```python
from build123d import *

# Parameters (mm, degrees)
F0_R     = 381
F1_DEPTH = 762
F3_W     = 50
F3_H     = 50
F3_W_2   = 40
F3_H_2   = 40
F4_DEPTH = 30
F5_W     = 50
F5_H     = 50
F5_W_2   = 40
F5_H_2   = 40
F6_DEPTH = 30
F7_SIZE  = 24.99999


# Not quite as in the source:
# - a fillet or chamfer is up to 0.001 mm smaller than in the source, because OpenCascade refuses the exact size


with BuildPart() as f1:
    # F0 (on Top) → F1 (new body)
    with BuildSketch(Plane.XY):
        Circle(F0_R)
    extrude(amount=F1_DEPTH)


with BuildPart() as f4:
    # F3 (on Top) → F4 (new body)
    with BuildSketch(Plane.XY):
        Rectangle(F3_W, F3_H)
        Rectangle(F3_W_2, F3_H_2, mode=Mode.SUBTRACT)
    extrude(amount=F4_DEPTH)

    # F5 (on face) → F6 (join)
    with BuildSketch(Plane.XY.offset(30)):
        Rectangle(F5_W, F5_H)
        Rectangle(F5_W_2, F5_H_2, mode=Mode.SUBTRACT)
        Rectangle(F5_W_2, F5_H_2)
    extrude(amount=F6_DEPTH)

    # F7 (size 25 in the source; OpenCascade refuses exactly that, so slightly less here)
    f7_edges = [f4.edges().sort_by_distance(p)[0] for p in [
        (25, 0, 60),
        (0, 25, 60),
        (-25, 0, 60),
        (0, -25, 60),
    ]]
    chamfer(f7_edges, length=F7_SIZE)


solid = f4.part
```
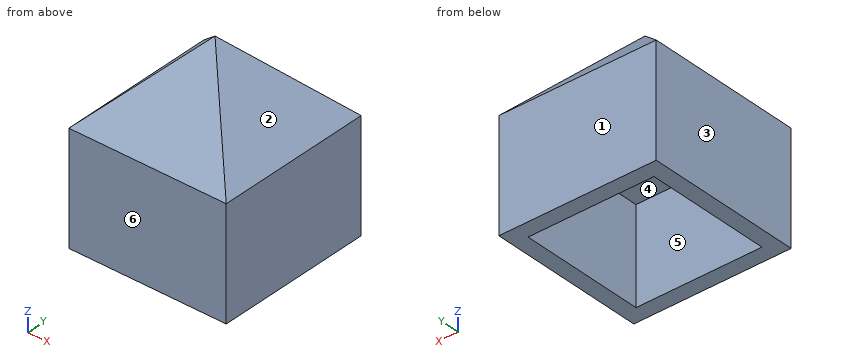
Source: CAD feature listing. Evaluate the final solid. Frame: model axes, mm. Face numbers are marked on the shaded views. A direction names the side the tool comes from. Give positions to 0.01 mm unless a question says otherwise; leave off trailing zeros. Write each loop counter-clockwise with the first axis right and the second up, starting at its lowest first coordinate (ties: lowest second). Pieces come first, ordered by that corner, then holes. Notation, with made-up numbers: (40, 47) - (79, 47) arc R14 cw to (79, 64) - close; hole circle Ø10 at (49.5, 71.25). An arc over 180 degrees is marked (long way). One line per item, written item: value. Start each with the question number.
Q1. Set-up query: the marked faces 5 and 6. Return all of +Z, -Z, +X, -X, +Y, -Y with unobstructed straight access to the full face (end or side cutting, diameter ignored); none if empty.
Q2. Material intervals for probe 1 along Y at (x, z) = (-16, 26.5); probe 2 along Z at (x, y) = (-16, 6.5), sorted ascending. Write a range as from..to.
Q3. Section query D-D, the plane z = 39. Return the cut outline in (x, y), then the cut area to 3 significant figures.
Q4. Section query A-A, the plane z = 12.5. Return the cut outline in (x, y), then the cut area to 3 significant figures.
Q5. Section query B-B, the plane x = -6.5. Return the cut outline in (y, z).
Q6. Section query C-C, the plane y = -6. Return the cut outline in (x, z), then the cut area to 3 significant figures.
Q7. First-contact query: pin 1 Ø4 at (y, z) = (6.5, 47.5) entering from +X; pin 2 Ø12 at (x, y) = (-5, 6.5) entering from -Z; pin 3 Ø4 at (y, z) = (-3.5, 48) entering from -X. Flat tips, straight axial feed; report the tip coordinate or a pass-through.
Q8. Draft query along X for the marked faces 1, 2, 3 and 4. Return one class per face: +X half, -X half, draft (parallel to the pull), parting line (faces both ways), or undercut.
Answer:
1. face 5: -Z
1. face 6: +Z, -Z, +X, -X, -Y
2. probe 1: y = -25..-20, 20..25
2. probe 2: z = 30..44
3. outline: (-21, -21) - (21, -21) - (21, 21) - (-21, 21) - close
3. area: 1,760 mm2
4. outline: (-25, -25) - (25, -25) - (25, 25) - (-25, 25) - close; hole (-20, -20) - (20, -20) - (20, 20) - (-20, 20) - close
4. area: 900 mm2
5. outline: (-25, 0) - (-20, 0) - (-20, 30) - (20, 30) - (20, 0) - (25, 0) - (25, 35) - (6.5, 53.5) - (-6.5, 53.5) - (-25, 35) - close
6. outline: (-25, 0) - (-20, 0) - (-20, 30) - (20, 30) - (20, 0) - (25, 0) - (25, 35) - (6, 54) - (-6, 54) - (-25, 35) - close
6. area: 1,140 mm2
7. pin 1: stops at x = 14.5
7. pin 2: stops at z = 30
7. pin 3: stops at x = -14
8. face 1: draft
8. face 2: +X half
8. face 3: -X half
8. face 4: undercut
